from build123d import *

# Parameters (mm, degrees)
BOSS_EXTRU_1_DEPTH      = 4
BOSS_EXTRU_3_DEPTH      = 35
ESQUISSE2_R             = 3
BOSS_EXTRU_2_DEPTH      = 3
ENL_V_MAT_EXTRU_1_REACH = 129.501
CONG_1_R                = 2
ESQUISSE7_R             = 4
ESQUISSE7_R_2           = 1.5
ESQUISSE7_R_3           = 2
BOSS_EXTRU_5_DEPTH      = 30


with BuildPart() as part:
    # Esquisse1 → Boss.-Extru.1 (new body)
    with BuildSketch(Plane.XY):
        with BuildLine():
            Line((54.5, 0), (-54.5, 0))
            ThreePointArc((-54.5, 0), (-64.919772429, 33.614061701), (-36.233707498, 54))
            ThreePointArc((-36.233707498, 54), (-4.477813337, 79.931662315), (23.49840511, 49.96135825))
            ThreePointArc((23.49840511, 49.96135825), (47.514151238, 49.231040909), (53.49840511, 25.96135825))
            ThreePointArc((53.49840511, 25.96135825), (66.48874108, 13.462528258), (54.5, 0))
        make_face()
    extrude(amount=BOSS_EXTRU_1_DEPTH)

    # Esquisse4 → Boss.-Extru.3 (add)
    with BuildSketch(Plane.XY):
        with BuildLine():
            Line((-55.473558679, -3), (54.609729917, -3))
            ThreePointArc((54.609729917, -3), (69.434198001, 11.529399821), (57.437462173, 28.468899301))
            ThreePointArc((57.437462173, 28.468899301), (49.838372291, 51.204095649), (26.142843315, 54.831384802))
            ThreePointArc((26.142843315, 54.831384802), (-5.438581775, 82.982875193), (-38.767146442, 56.92333569))
            ThreePointArc((-38.767146442, 56.92333569), (-68.289321366, 32.863500835), (-55.473558679, -3))
        make_face()
        with BuildLine():
            Line((-54.5, 0), (54.5, 0))
            ThreePointArc((54.5, 0), (66.48874108, 13.462528258), (53.49840511, 25.96135825))
            ThreePointArc((53.49840511, 25.96135825), (47.514151238, 49.231040909), (23.49840511, 49.96135825))
            ThreePointArc((23.49840511, 49.96135825), (-4.477813337, 79.931662315), (-36.233707498, 54))
            ThreePointArc((-36.233707498, 54), (-64.919772429, 33.614061701), (-54.5, 0))
        make_face(mode=Mode.SUBTRACT)
    extrude(amount=BOSS_EXTRU_3_DEPTH)

    # Esquisse2 → Boss.-Extru.2 (add)
    # profile 1 of 3: a face of its own
    with BuildSketch(Plane.XY):
        with BuildLine():
            Line((-47, -3), (-47, -15))
            ThreePointArc((-47, -15), (-41, -21), (-35, -15))
            Line((-35, -15), (-35, -3))
            Line((-35, -3), (-47, -3))
        make_face()
        with Locations((-41, -15)):
            Circle(ESQUISSE2_R, mode=Mode.SUBTRACT)
    # profile 2 of 3: a face of its own
    with BuildSketch(Plane.XY):
        with BuildLine():
            Line((35, -15), (35, -3))
            Line((35, -3), (47, -3))
            Line((47, -3), (47, -15))
            ThreePointArc((47, -15), (41, -21), (35, -15))
        make_face()
        with Locations(Location((41, -15, 0), (0, 0, 180))):
            Circle(ESQUISSE2_R, mode=Mode.SUBTRACT)
    # profile 3 of 3: a face of its own
    with BuildSketch(Plane.XY):
        with BuildLine():
            Line((-14, 82.136794295), (-14, 92))
            ThreePointArc((-14, 92), (-8, 98), (-2, 92))
            Line((-2, 92), (-2, 82.691525928))
            ThreePointArc((-2, 82.691525928), (-8.025454596, 82.964796006), (-14, 82.136794295))
        make_face()
        with Locations((-8, 92)):
            Circle(ESQUISSE2_R, mode=Mode.SUBTRACT)
    extrude(amount=BOSS_EXTRU_2_DEPTH)

    # Esquisse6 → Enlèv. mat.-Extru.1 (cut, up to next)
    with BuildSketch(Plane.XZ.offset(3), mode=Mode.PRIVATE) as enl_v_mat_extru_1_sk1:
        with BuildLine():
            Line((2.455969349, 12), (-2.455969349, 12))
            ThreePointArc((-2.455969349, 12), (-2.499533293, 12.003179881), (-2.542173715, 12.012652114))
            Line((-2.542173715, 12.012652114), (-4.786204366, 12.68586131))
            ThreePointArc((-4.786204366, 12.68586131), (-4.940687878, 12.794130036), (-5, 12.973209195))
            Line((-5, 12.973209195), (-5, 13.2))
            ThreePointArc((-5, 13.2), (-4.912132034, 13.412132034), (-4.7, 13.5))
            Line((-4.7, 13.5), (4.7, 13.5))
            ThreePointArc((4.7, 13.5), (4.912132034, 13.412132034), (5, 13.2))
            Line((5, 13.2), (5, 12.973209195))
            ThreePointArc((5, 12.973209195), (4.940687878, 12.794130036), (4.786204366, 12.68586131))
            Line((4.786204366, 12.68586131), (2.542173715, 12.012652114))
            ThreePointArc((2.542173715, 12.012652114), (2.499533293, 12.003179881), (2.455969349, 12))
        make_face()
    enl_v_mat_extru_1_tool1 = extrude(enl_v_mat_extru_1_sk1.sketch, amount=-ENL_V_MAT_EXTRU_1_REACH, mode=Mode.PRIVATE) & part.part
    add(enl_v_mat_extru_1_tool1.solids().sort_by_distance((0, -3, 12.819686))[0], mode=Mode.SUBTRACT)

    # Congé1
    cong_1_edges = [part.edges().sort_by_distance(p)[0] for p in [
        (-41, -3, 3),
        (-35, -3, 1.5),
        (-47, -3, 1.5),
        (-8.025454596, 82.964796006, 3),
        (-14, 82.136794295, 1.5),
        (-2, 82.691525928, 1.5),
        (41, -3, 3),
        (47, -3, 1.5),
        (35, -3, 1.5),
    ]]
    fillet(cong_1_edges, radius=CONG_1_R)

    # Esquisse7 → Boss.-Extru.5 (add)
    # profile 1 of 3: a face of its own
    with BuildSketch(Plane.XY):
        with Locations((0, 77.234712914)):
            Circle(ESQUISSE7_R)
        with Locations((0, 77.234712914)):
            Circle(ESQUISSE7_R_2, mode=Mode.SUBTRACT)
    # profile 2 of 3: a face of its own
    with BuildSketch(Plane.XY):
        with Locations((-64, 24)):
            Circle(ESQUISSE7_R)
        with Locations((-64, 24)):
            Circle(ESQUISSE7_R_3, mode=Mode.SUBTRACT)
    # profile 3 of 3: a face of its own
    with BuildSketch(Plane.XY):
        with Locations((64, 12)):
            Circle(ESQUISSE7_R)
        with Locations((64, 12)):
            Circle(ESQUISSE7_R_3, mode=Mode.SUBTRACT)
    extrude(amount=BOSS_EXTRU_5_DEPTH)


solid = part.part
Here's how the part is built. I have some questions about the finished solid (model axes, mm). A direction names the side the tool comes from. Coordinates: 2 decimals unless noted, no trailing zeros. Write each loop counter-clockwise with the first axis right and the second up, starting at its lowest first coordinate (ties: lowest second). Pieces come first, ordered by that corner, then holes.
1) Thinking about a two-plate mould opening in Z: for faces 4 (the face through (0, 77, 4)), 5 (the face through (43.4, -13.2, 1.5)), 6 (the face through (0, -2, 13.5)), which applies, +Z half, -Z half, draft (parallel to the pull), parting line (faces both ways), or undercut?
Filled in:
face 4: +Z half
face 5: draft
face 6: undercut
2) If we section it at B-B (x = 41): List the corners of the cut face in (y, z) for me, plus the area to 3 significant figures.
Filled in:
outline: (-21, 0) - (-18, 0) - (-18, 3) - (-21, 3) - close; (-12, 0) - (55.82, 0) - (55.82, 35) - (52.7, 35) - (52.7, 4) - (0, 4) - (0, 35) - (-3, 35) - (-3, 5) arc R2 cw to (-5, 3) - (-12, 3) - close
area: 462 mm2
3) If I drill on line 1 (X direction, y = 24, z = 13); line 2 (Y direction, x = 64, z = 21); line 3 (Z direction, x = 31, y = 28), over which ranges is the centre line in solid material (lowest first)?
Filled in:
line 1: x = -69.5 to -66, -62 to -60, 60.36 to 65.08
line 2: y = 0.89 to 5.3, 8 to 10, 14 to 16, 20.62 to 25.03
line 3: z = 0 to 4
4) Which directions (+Z, -Z, +X, -X, +Y, -Y) give clear straight access to the entire face, cutting with the end or side of a thin tool? Please do faces 1 (the face through (64, 14, 17)), 2 (the face through (-8, 88, 3)), 3 (the face through (-41, -11, 3)).
Filled in:
face 1: +Z
face 2: +Z, +X, -X, +Y
face 3: +Z, +X, -X, -Y
5) I'm going to push flat-ended pins straight in: pin 1 (6 mm diameter, centred on x = 42.5, y = -15, fed in from +Z); pin 2 (2 mm diameter, centred on x = 28, y = 39, fed in from +Z); pin 3 (8 mm diameter, centred on x = 8, z = 25, fed in from +Y); pin 4 (3.5 mm diameter, centred on x = -8, y = 92, fed in from -Z). Where does each tip first touch, or does it pass through?
Filled in:
pin 1: stops at z = 3
pin 2: stops at z = 4
pin 3: stops at y = 81.28
pin 4: passes through
6) If we section it at A-A (z = 33): List the corners of the cut face in (x, y) for me, plus the area to 3 significant figures.
Filled in:
outline: (-55.47, -3) - (54.61, -3) arc R16 ccw to (57.44, 28.47) arc R23 ccw to (26.14, 54.83) arc R33 ccw to (-38.77, 56.92) arc R33 ccw to start; hole (-54.5, 0) - (54.5, 0) arc R13 ccw to (53.5, 25.96) arc R20 ccw to (23.5, 49.96) arc R30 ccw to (-36.23, 54) arc R30 ccw to start
area: 1,120 mm2
7) If we section it at D-D (x = -18): List the corners of the cut face in (y, z) for me, plus the area to 3 significant figures.
Filled in:
outline: (-3, 0) - (80.93, 0) - (80.93, 35) - (77.71, 35) - (77.71, 4) - (0, 4) - (0, 35) - (-3, 35) - close
area: 529 mm2
8) If we section it at C-C (z = 22.5): List the corners of the cut face in (x, y) for me, plus the area to 3 significant figures.
Filled in:
outline: (-55.47, -3) - (54.61, -3) arc R16 ccw to (57.44, 28.47) arc R23 ccw to (26.14, 54.83) arc R33 ccw to (-38.77, 56.92) arc R33 ccw to start; hole (-66.32, 20.74) arc R30 ccw to (-54.5, 0) - (54.5, 0) arc R13 ccw to (65.66, 8.36) arc R4 cw (long way) to (66.29, 15.28) arc R13 ccw to (53.5, 25.96) arc R20 ccw to (23.5, 49.96) arc R30 ccw to (3.9, 78.14) arc R4 cw (long way) to (-3.07, 79.8) arc R30 ccw to (-36.23, 54) arc R30 ccw to (-66.32, 27.26) arc R4 cw (long way) to start; hole circle Ø4 at (-64, 24); hole circle Ø3 at (0, 77.23); hole circle Ø4 at (64, 12)
area: 1,210 mm2
